from build123d import *

# Parameters (mm, degrees)
F1_DEPTH = 2


with BuildPart() as f1:
    # F0 (on Top) → F1 (new body)
    with BuildSketch(Plane.XY):
        with BuildLine():
            Line((-13.021325, 16.75), (-19, 16.75))
            ThreePointArc((-19, 16.75), (-20.414214, 16.164214), (-21, 14.75))
            Line((-21, 14.75), (-21, -6.277864))
            ThreePointArc((-21, -6.277864), (-22.253198, -7.85105), (-22.91608, -9.75))
            Line((-22.91608, -9.75), (-20, -9.75))
            Line((-20, -9.75), (-20, -11.75))
            Line((-20, -11.75), (-22.91608, -11.75))
            ThreePointArc((-22.91608, -11.75), (-20.872983, -15.332576), (-17, -16.75))
            Line((-17, -16.75), (-17, -0.25))
            Line((-17, -0.25), (-15, -0.25))
            Line((-15, -0.25), (-15, -16.75))
            Line((-15, -16.75), (15, -16.75))
            Line((15, -16.75), (15, -0.25))
            Line((15, -0.25), (17, -0.25))
            Line((17, -0.25), (17, -16.75))
            ThreePointArc((17, -16.75), (20.872983, -15.332576), (22.91608, -11.75))
            Line((22.91608, -11.75), (20, -11.75))
            Line((20, -11.75), (20, -9.75))
            Line((20, -9.75), (22.91608, -9.75))
            ThreePointArc((22.91608, -9.75), (22.253198, -7.85105), (21, -6.277864))
            Line((21, -6.277864), (21, 14.75))
            ThreePointArc((21, 14.75), (20.414214, 16.164214), (19, 16.75))
            Line((19, 16.75), (13.021325, 16.75))
            ThreePointArc((13.021325, 16.75), (11.948416, 16.437859), (11.210407, 15.598868))
            Line((11.210407, 15.598868), (8.539593, 9.901132))
            ThreePointArc((8.539593, 9.901132), (7.801584, 9.062141), (6.728675, 8.75))
            Line((6.728675, 8.75), (-6.728675, 8.75))
            ThreePointArc((-6.728675, 8.75), (-7.801584, 9.062141), (-8.539593, 9.901132))
            Line((-8.539593, 9.901132), (-11.210407, 15.598868))
            ThreePointArc((-11.210407, 15.598868), (-11.948416, 16.437859), (-13.021325, 16.75))
        make_face()
    extrude(amount=F1_DEPTH)


solid = f1.part
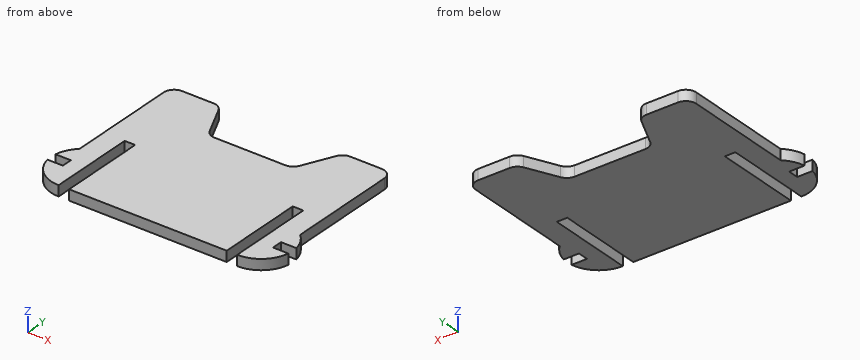
Could you check a few things on this model? Use its own coordinates, in mm. Give positions to 0.01 mm unless a question says otherwise; leave off trailing zeros. Order: outer loops, then holes, each group sorted by start corner. A loop starts at its lowest first (then second) coordinate and runs counter-clockwise, first axis right, second up.
1. Suppose I cut it at D-D (x = -9.5). Write out the boundary of the cut face in (y, z), plus the area to 3 significant figures.
Answers below:
outline: (-16.75, 0) - (11.95, 0) - (11.95, 2) - (-16.75, 2) - close
area: 57.4 mm2
2. Suppose I cut it at C-C (y = 10.5). Write out the boundary of the cut face in (x, z), plus the area to 3 significant figures.
Answers below:
outline: (-21, 0) - (-8.82, 0) - (-8.82, 2) - (-21, 2) - close; (8.82, 0) - (21, 0) - (21, 2) - (8.82, 2) - close
area: 48.7 mm2
3. I need wall thicknesses on L1, parallel to X at y = -10.5, z = 0.8; L2, parallel to X at y = -13, z = 1.05; L3, parallel to Y at x = 4.5, z = 0.95. Which ranges of each line are inside material? Lowest first, please.
Answers below:
L1: x = -20 to -17, -15 to 15, 17 to 20
L2: x = -22.56 to -17, -15 to 15, 17 to 22.56
L3: y = -16.75 to 8.75
4. Suppose I cut it at A-A (y = -1.5). Write out the boundary of the cut face in (x, z), plus the area to 3 significant figures.
Answers below:
outline: (-21, 0) - (-17, 0) - (-17, 2) - (-21, 2) - close; (-15, 0) - (15, 0) - (15, 2) - (-15, 2) - close; (17, 0) - (21, 0) - (21, 2) - (17, 2) - close
area: 76.0 mm2
5. For pin 1 (1 mm diameter, centred on y = -10.5, z = 1.5, fed in from +X); pin 2 (1 mm diameter, centred on y = -8, z = 1.5, fed in from -X); pin 3 (1 mm diameter, centred on y = 1.5, z = 1.5, fed in from -X), each with a flat end and sliding along its axis, tell me the tip position at first contact or that it passes through.
Answers below:
pin 1: stops at x = 20
pin 2: stops at x = -22.56
pin 3: stops at x = -21
